from build123d import *

# Parameters (mm, degrees)
PAD_DEPTH       = 10
POCKET_DEPTH    = 3
SKETCH002_W     = 5.905023
SKETCH002_H     = 16.995962
SKETCH002_W_2   = 5.877612
SKETCH002_H_2   = 17.170593
SKETCH002_W_3   = 6.373988
POCKET001_DEPTH = 10.001
PAD001_DEPTH    = 5


with BuildPart() as part:
    # Sketch → Pad (new body)
    with BuildSketch(Plane.XY):
        Polygon((-20, 50), (20, 50), (40, 20), (20, -10), (20, -30), (-20, -30), (-20, -10), (-40, 20), align=None)
    extrude(amount=PAD_DEPTH)

    # Sketch001 (on Face10 of Pad) → Pocket (cut)
    with BuildSketch(Plane.XY.offset(10)):
        Polygon((-15.351509, 30), (-20, 20), (-10, 20), align=None)
        Polygon((10, 20), (20, 20), (15.157187, 30), align=None)
    extrude(amount=-POCKET_DEPTH, mode=Mode.SUBTRACT)

    # Sketch002 (on Face5 of Pocket) → Pocket001 (cut, through all)
    with BuildSketch(Plane.XY.offset(10)):
        with Locations((-12.952511, -18.497981)):
            Rectangle(SKETCH002_W, SKETCH002_H)
        with Locations((12.938806, -18.585296)):
            Rectangle(SKETCH002_W_2, SKETCH002_H_2)
        with Locations((0.029951, -18.585296)):
            Rectangle(SKETCH002_W_3, SKETCH002_H_2)
    extrude(amount=-POCKET001_DEPTH, mode=Mode.SUBTRACT)

    # Sketch003 (on Face5 of Pocket001) → Pad001 (join)
    with BuildSketch(Plane.XY.offset(10)):
        Polygon((0, 16.734911), (-5.724616, 6.843517), (5.68853, 6.784989), align=None)
    extrude(amount=PAD001_DEPTH)


solid = part.part
Geometry: final body of the model. Coordinates: model frame, mm. A direction names the side the tool comes from. Round coordinates to 2 decimals unless told otherwise and drop trailing zeros. Loops run counter-clockwise (first coordinate to the right, second up) from the corner with the lowest first, then second, coordinate; pieces in that order, holes last. Notation, with made-up numbers: M 20,80.25 L 61,80.25 A28 cw 61,110.25 Z; hole C 55.25,-12.75 d2. An arc over 180 degrees is marked long. One line per question, with ' | ' between items.
(1) Pull-direction query (Y, two-part tool) for faces 6 (the flat face through (1, 19, 10)), 7 (the flat face through (0, -30, 5)), 8 (the flat face through (-17.643, 25.07, 8.521)); classes: +Y half, -Y half, draft (parallel to the pull), parting line (faces both ways), or undercut.
Check result:
face 6: draft | face 7: -Y half | face 8: undercut
(2) Cut plane C-C on x = -2. Return the cut outline in (y, z).
Check result:
outline: M -30,0 L -27.17,0 L -27.17,10 L -30,10 Z; M -10,0 L 50,0 L 50,10 L 13.28,10 L 13.28,15 L 6.82,15 L 6.82,10 L -10,10 Z
(3) Material intervals for line 1 along X through (y, z) = (-11.5, 1); line 2 along X through (y, z) = (28, 7.75); line 3 along Y through (x, z) = (-3, 1.5), sorted ascending. Write a range as from..to.
Check result:
line 1: x = -20..-15.91, -10..-3.16, 3.22..10, 15.88..20 | line 2: x = -34.67..-16.28, -14.28..14.13, 16.13..34.67 | line 3: y = -30..-27.17, -10..50
(4) Cut plane B-B on z = 5.5. Return the cut outline in (x, y), plus the area to 3 significant figures.
Check result:
outline: M -40,20 L -20,-10 L -20,-30 L 20,-30 L 20,-10 L 40,20 L 20,50 L -20,50 Z; hole M -15.91,-27 L -10,-27 L -10,-10 L -15.91,-10 Z; hole M -3.16,-27.17 L 3.22,-27.17 L 3.22,-10 L -3.16,-10 Z; hole M 10,-27.17 L 15.88,-27.17 L 15.88,-10 L 10,-10 Z | area: 4,090 mm2
(5) Cut plane A-A on y = -18. Return the cut outline in (x, z), plus the area to 3 significant figures.
Check result:
outline: M -20,0 L -15.91,0 L -15.91,10 L -20,10 Z; M -10,0 L -3.16,0 L -3.16,10 L -10,10 Z; M 3.22,0 L 10,0 L 10,10 L 3.22,10 Z; M 15.88,0 L 20,0 L 20,10 L 15.88,10 Z | area: 218 mm2
(6) Access query for faces 1 (the flat face through (2.884, 11.69, 12.465)), 2 (the flat face through (12.615, 25.07, 8.521)), 3 (the flat face through (-13, -26.996, 5)), 4 (the flat face through (20, -20, 5)), 5 (the flat face through (-20, -20, 5)). Directions: +Z, -Z, +X, -X, +Y, -Y. A direction counts if a zero-diameter tool reaches every point of the face in a straight line with its end or side. Return the directions, or none.
Check result:
face 1: +Z, +X, +Y | face 2: +Z | face 3: +Z, -Z | face 4: +Z, -Z, +X, -Y | face 5: +Z, -Z, -X, -Y
(7) Contact query for flat-ended pins moving along their axis: P1, Ø3, axis at y = -22.5, z = 5.5, coming from the +X side; P2, Ø1, axis at x = 22.5, y = -4, coming from the -Z side; P3, Ø2, axis at y = 4, z = 2.5, coming from the +X side; P4, Ø5, axis at y = -22, z = 2.5, coming from the -X side. Output: stop coordinate, or through.
Check result:
P1: stops at x = 20 | P2: stops at z = 0 | P3: stops at x = 30 | P4: stops at x = -20
(8) Cut plane D-D on x = -23.5. Return the cut outline in (y, z), plus the area to 3 significant figures.
Check result:
outline: M -4.75,0 L 44.75,0 L 44.75,10 L -4.75,10 Z | area: 495 mm2
